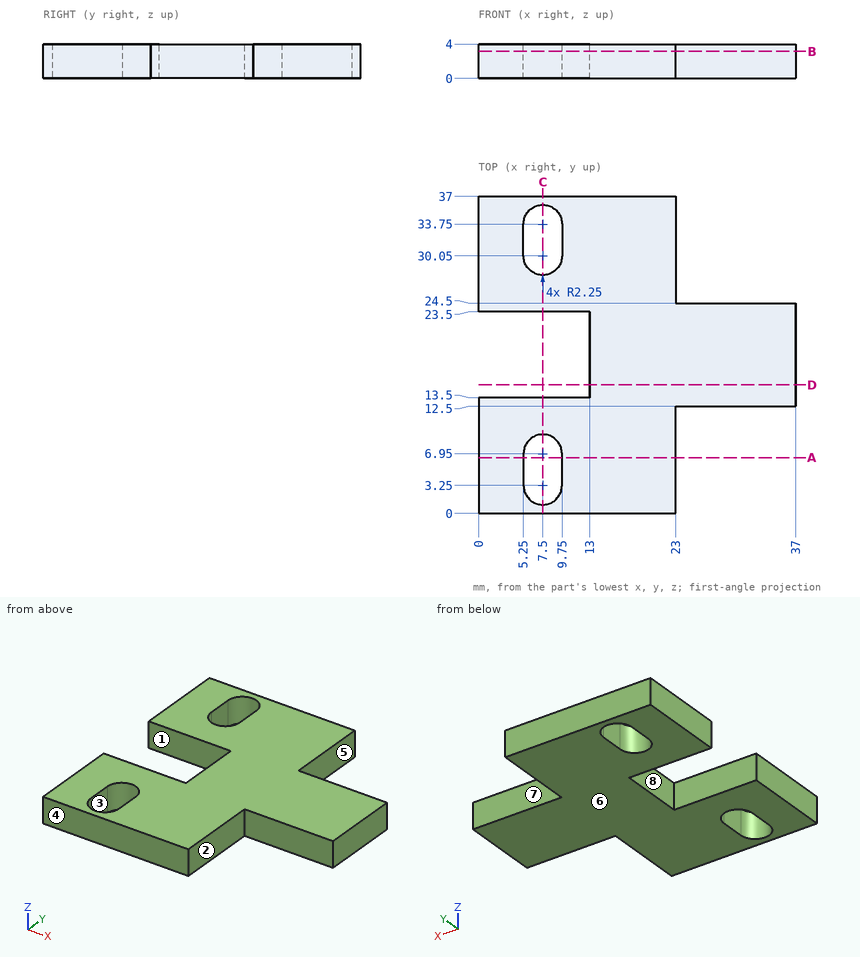
The figure shows three views and two pictorial views of one solid part (mm, origin at its lowest corner). Answer the questions. A direction names the side the tool comes from. Round coordinates to 2 decimals unless told otherwise and drop trailing zeros. Order: outer loops, then holes, each group sorted by start corner. A loop starts at its lowest first (then second) coordinate and runs counter-clockwise, first axis right, second up. Notation, with made-up numbers: (60, 26) - (113, 26) arc R17 ccw to (113, 38) - close; hole circle Ø7 at (-21.75, -38). An arc over 180 degrees is marked (long way). Write item = value, one per line. Start each with the question number.
1) Section A-A, the plane y = 6.5 is taken. Write down the section's boundary in (x, z), plus the area to 3 significant figures.
2) Straight lines are drawn through the part: L1, parallel to X at y = 33, z = 1.2; L2, parallel to Y at x = 10.5, z = 3.7; L3, parallel to X at y = 12, z = 0.8. For each, find the intervals that lie inside material, in ascending order.
3) For the marked faces 1, 2, 3, 4 and 5, determine the directions among +Z, -Z, +X, -X, +Y, -Y from which every point of the face is accessible in a straight line to the end or side of a thin tool.
4) Section D-D, the plane y = 15 is taken. Write down the section's boundary in (x, z), plus the area to 3 significant figures.
5) Section B-B, the plane z = 3.15 is taken. Write down the section's boundary in (x, y).
6) Section C-C, the plane x = 7.5 is taken. Write down the section's boundary in (y, z), plus the area to 3 significant figures.
7) Given pin 1 (1.1 mm diameter, centred on y = 5.5, z = 3, fed in from +X), flat-ended and moving along its own axis, determine where the tip first touches the part or whether it passes through.
8) For a pull along Y with two mould halves and no side action, classify the marked faces 6, 7 and 8 as released by +Y, released by -Y, zero draft, split by the parting line, or undercut.
Results list:
q1.outline = (0, 0) - (5.25, 0) - (5.25, 4) - (0, 4) - close; (9.75, 0) - (23, 0) - (23, 4) - (9.75, 4) - close
q1.area = 74.0 mm^2
q2.L1 = 0 to 5.25, 9.75 to 23
q2.L2 = 0 to 13.5, 23.5 to 37
q2.L3 = 0 to 23
q3.face_1 = +Z, -Z, -X
q3.face_2 = +Z, -Z, +X, -Y
q3.face_3 = +Z, -Z
q3.face_4 = +Z, -Z, +X, -X, -Y
q3.face_5 = +Z, -Z, +X, +Y
q4.outline = (13, 0) - (37, 0) - (37, 4) - (13, 4) - close
q4.area = 96.0 mm^2
q5.outline = (0, 0) - (23, 0) - (23, 12.5) - (37, 12.5) - (37, 24.5) - (23, 24.5) - (23, 37) - (0, 37) - (0, 23.5) - (13, 23.5) - (13, 13.5) - (0, 13.5) - close; hole (5.25, 3.25) arc R2.25 ccw to (9.75, 3.25) - (9.75, 6.95) arc R2.25 ccw to (5.25, 6.95) - close; hole (5.25, 30.05) arc R2.25 ccw to (9.75, 30.05) - (9.75, 33.75) arc R2.25 ccw to (5.25, 33.75) - close
q6.outline = (0, 0) - (1, 0) - (1, 4) - (0, 4) - close; (9.2, 0) - (13.5, 0) - (13.5, 4) - (9.2, 4) - close; (23.5, 0) - (27.8, 0) - (27.8, 4) - (23.5, 4) - close; (36, 0) - (37, 0) - (37, 4) - (36, 4) - close
q6.area = 42.4 mm^2
q7.pin_1 = 23
q8.face_6 = zero draft
q8.face_7 = released by +Y
q8.face_8 = undercut
